```python
from build123d import *

# Parameters (mm, degrees)
SKETCH1_R                                       = 12.446
SKETCH1_R_2                                     = 1.27
BOSS_EXTRUDE1_DEPTH                             = 24.892
CSK_FOR_M3_FLAT_HEAD_MACHINE_SCREW1_D           = 3.4
CSK_FOR_M3_FLAT_HEAD_MACHINE_SCREW1_CSINK_D     = 6.3
CSK_FOR_M3_FLAT_HEAD_MACHINE_SCREW1_CSINK_ANGLE = 90
SKETCH5_R                                       = 12.192
BOSS_EXTRUDE2_DEPTH                             = 30.734
SKETCH6_R                                       = 3.556
BOSS_EXTRUDE3_DEPTH                             = 2.54
SKETCH7_R                                       = 2.032
BOSS_EXTRUDE4_DEPTH                             = 9.906
SKETCH8_W                                       = 2.032
SKETCH8_H                                       = 0.254
CUT_EXTRUDE2_DEPTH                              = 9.906
SKETCH9_R                                       = 3.175
BOSS_EXTRUDE5_DEPTH                             = 1.524
SKETCH10_W                                      = 2.032
SKETCH10_H                                      = 0.254
BOSS_EXTRUDE6_DEPTH                             = 4.318
SKETCH11_R                                      = 11.557
SKETCH11_W                                      = 2.032
SKETCH11_H                                      = 0.254
BOSS_EXTRUDE7_DEPTH                             = 0.508
SKETCH12_W                                      = 12.7
SKETCH12_H                                      = 5.08
BOSS_EXTRUDE8_DEPTH                             = 2.54
SKETCH13_W                                      = 3.81
SKETCH13_H                                      = 2.54
BOSS_EXTRUDE9_DEPTH                             = 2.794
BOSS_EXTRUDE10_DEPTH                            = 9.652
SKETCH15_R                                      = 3.175
BOSS_EXTRUDE11_DEPTH                            = 0.508
SKETCH16_R                                      = 6.985
BOSS_EXTRUDE12_DEPTH                            = 6.35


with BuildPart() as part:
    # Sketch1 → Boss-Extrude1 (new body)
    with BuildSketch(Plane(origin=(0, 0, 0), x_dir=(1, 0, 0), z_dir=(0, 1, 0))):
        Circle(SKETCH1_R)
        with Locations((-9.017, 0)):
            Circle(SKETCH1_R_2, mode=Mode.SUBTRACT)
        with Locations((9.017, 0)):
            Circle(SKETCH1_R_2, mode=Mode.SUBTRACT)
    extrude(amount=BOSS_EXTRUDE1_DEPTH)

    # CSK for M3 Flat Head Machine Screw1 (through all)
    with Locations(Plane(origin=(0, 24.892, 0), x_dir=(1, 0, 0), z_dir=(0, 1, 0))):
        with Locations((0, 8.119865968), (0, -7.587036194)):
            CounterSinkHole(CSK_FOR_M3_FLAT_HEAD_MACHINE_SCREW1_D / 2, CSK_FOR_M3_FLAT_HEAD_MACHINE_SCREW1_CSINK_D / 2, counter_sink_angle=CSK_FOR_M3_FLAT_HEAD_MACHINE_SCREW1_CSINK_ANGLE)

    # Sketch5 → Boss-Extrude2 (add)
    with BuildSketch(Plane(origin=(0, 24.892, 0), x_dir=(1, 0, 0), z_dir=(0, 1, 0))):
        Circle(SKETCH5_R)
    extrude(amount=BOSS_EXTRUDE2_DEPTH)

    # Sketch6 → Boss-Extrude3 (add)
    with BuildSketch(Plane(origin=(0, 0, 0), x_dir=(1, 0, 0), z_dir=(0, 1, 0))):
        Circle(SKETCH6_R)
    extrude(amount=-BOSS_EXTRUDE3_DEPTH)

    # Sketch7 → Boss-Extrude4 (add)
    with BuildSketch(Plane(origin=(0, -2.54, 0), x_dir=(-1, 0, 0), z_dir=(0, -1, 0))):
        Circle(SKETCH7_R)
    extrude(amount=BOSS_EXTRUDE4_DEPTH)

    # Sketch8 → Cut-Extrude2 (cut)
    with BuildSketch(Plane(origin=(0, -12.446, 0), x_dir=(-1, 0, 0), z_dir=(0, -1, 0))):
        with Locations((0, -1.905)):
            Rectangle(SKETCH8_W, SKETCH8_H)
        with Locations((0, 1.905)):
            Rectangle(SKETCH8_W, SKETCH8_H)
    extrude(amount=-CUT_EXTRUDE2_DEPTH, mode=Mode.SUBTRACT)

    # Sketch9 → Boss-Extrude5 (add)
    with BuildSketch(Plane(origin=(0, 55.626, 0), x_dir=(1, 0, 0), z_dir=(0, 1, 0))):
        Circle(SKETCH9_R)
    extrude(amount=BOSS_EXTRUDE5_DEPTH)

    # Sketch10 → Boss-Extrude6 (add)
    with BuildSketch(Plane(origin=(0, 55.626, 0), x_dir=(1, 0, 0), z_dir=(0, 1, 0))):
        with Locations((-9.017, 0)):
            Rectangle(SKETCH10_W, SKETCH10_H)
        with Locations((9.017, 0)):
            Rectangle(SKETCH10_W, SKETCH10_H)
    extrude(amount=BOSS_EXTRUDE6_DEPTH)

    # Sketch11 → Boss-Extrude7 (add)
    with BuildSketch(Plane(origin=(0, 57.15, 0), x_dir=(1, 0, 0), z_dir=(0, 1, 0))):
        Circle(SKETCH11_R)
        with Locations((-9.017, 0)):
            Rectangle(SKETCH11_W, SKETCH11_H, mode=Mode.SUBTRACT)
        with Locations((9.017, 0)):
            Rectangle(SKETCH11_W, SKETCH11_H, mode=Mode.SUBTRACT)
    extrude(amount=BOSS_EXTRUDE7_DEPTH)

    # Sketch12 → Boss-Extrude8 (add)
    with BuildSketch(Plane(origin=(0, 57.658, 0), x_dir=(1, 0, 0), z_dir=(0, 1, 0))):
        with Locations((0, 6.35)):
            Rectangle(SKETCH12_W, SKETCH12_H)
    extrude(amount=BOSS_EXTRUDE8_DEPTH)

    # Sketch13 → Boss-Extrude9 (add)
    with BuildSketch(Plane(origin=(0, 57.658, 0), x_dir=(1, 0, 0), z_dir=(0, 1, 0))):
        Rectangle(SKETCH13_W, SKETCH13_H)
    extrude(amount=BOSS_EXTRUDE9_DEPTH)

    # Sketch14 → Boss-Extrude10 (add)
    with BuildSketch(Plane(origin=(0, 57.658, 0), x_dir=(1, 0, 0), z_dir=(0, 1, 0))):
        Polygon((-5.718475067, -10.043071836), (5.597401443, -10.111050692), (5.615425354, -7.110759652), (-5.700451156, -7.042780797), align=None)
    extrude(amount=BOSS_EXTRUDE10_DEPTH)

    # Sketch15 → Boss-Extrude11 (add)
    with BuildSketch(Plane(origin=(0, 60.452, 0), x_dir=(1, 0, 0), z_dir=(0, 1, 0))):
        Circle(SKETCH15_R)
    extrude(amount=BOSS_EXTRUDE11_DEPTH)

    # Sketch16 → Boss-Extrude12 (add)
    with BuildSketch(Plane(origin=(0, 60.96, 0), x_dir=(1, 0, 0), z_dir=(0, 1, 0))):
        Circle(SKETCH16_R)
    extrude(amount=BOSS_EXTRUDE12_DEPTH)


solid = part.part
```
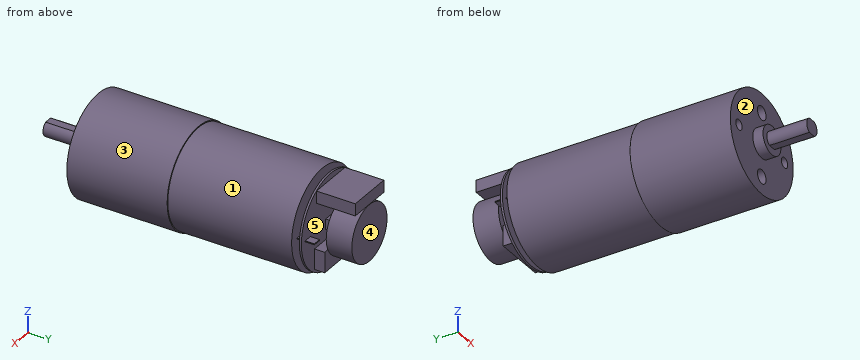
Verification items for the finished model (mm, model axes). Face numbers are marked on the shaded views. A direction names the side the tool comes from. Round coordinates to 2 decimals unless told otherwise and drop trailing zeros. Order: outer loops, then holes, each group sorted by start corner. A loop starts at its lowest first (then second) coordinate and runs counter-clockwise, first axis right, second up. Notation, with made-up numbers: (15, -5) - (41, -5) arc R21 cw to (41, 21) - close; hole circle Ø2 at (9.25, -10). An arc over 180 degrees is marked (long way). Use CSV: the item, a comma, the result in double quotes. Start each with the question number.
1) Section check A-A, the plane x = -4.5. Record the cut outline in (y, z).
2) Mould release check, pull along Z, two halves, no side actions. Record for the marked faces 3, 4 and 5: +Z half, -Z half, draft (parallel to the pull), parting line (faces both ways), or undercut.
3) Thickness scan on L1, parallel to Y at x = 3, z = -1.25; L2, parallel to Z at x = 0, y = 17.5; L3, parallel to X at y = 19.75, z = 0. Record the ranges inside material, lowest first.
4) Section check B-B, the plane y = -1.5. Record the cut outline in (x, z).
5) Go/stop test with flat-tipped pins: P1, Ø2, axis at x = -0.5, y = -6.5, coming from the +Z side; P2, Ø0.6, axis at x = -9.5, y = 59.5, coming from the +Z side; P3, Ø2, axis at x = -6, z = -0.5, coming from the -Y side. Record where each tip stops, or that it passes through.
6) Section check C-C, the plane x = 9. Record the cut outline in (y, z).
7) Access from +Z, -Z, +X, -X, +Y, -Y to the whole of each face (thin tool, end or side, straight path). Record for the marked faces 1 and 2.
Answers:
1,outline,"(0, -11.6) - (24.89, -11.6) - (24.89, -11.33) - (55.63, -11.33) - (55.63, 11.33) - (24.89, 11.33) - (24.89, 11.6) - (0, 11.6) - close; (57.15, -10.64) - (57.66, -10.64) - (57.66, -8.89) - (60.2, -8.89) - (60.2, -3.81) - (57.66, -3.81) - (57.66, 7.05) - (67.31, 7.05) - (67.31, 10.05) - (57.66, 10.05) - (57.66, 10.64) - (57.15, 10.64) - close; (60.96, -5.34) - (67.31, -5.34) - (67.31, 5.34) - (60.96, 5.34) - close"
2,face 3,"parting line"
2,face 4,"draft"
2,face 5,"undercut"
3,L1,"y = -2.54 to 55.63, 57.15 to 57.66, 60.96 to 67.31"
3,L2,"z = -12.45 to -9.82, -6.42 to 5.89, 9.29 to 12.45"
3,L3,"x = -12.45 to -10.29, -7.75 to 7.75, 10.29 to 12.45"
4,outline,"circle Ø7.11 at (0, 0)"
5,P1,"stops at z = 1.78"
5,P2,"stops at z = 0.13"
5,P3,"stops at y = 0"
6,outline,"(0, -8.6) - (24.89, -8.6) - (24.89, -8.22) - (55.63, -8.22) - (55.63, -0.13) - (57.15, -0.13) - (57.15, -7.25) - (57.66, -7.25) - (57.66, -0.13) - (59.94, -0.13) - (59.94, 0.13) - (57.66, 0.13) - (57.66, 7.25) - (57.15, 7.25) - (57.15, 0.13) - (55.63, 0.13) - (55.63, 8.22) - (24.89, 8.22) - (24.89, 8.6) - (0, 8.6) - (0, 1.27) - (24.89, 1.27) - (24.89, -1.27) - (0, -1.27) - close"
7,face 1,"+Y"
7,face 2,"-Y"
